For this review, use the dimensioned drawing (mm, ordinates from the lowest corner) and the shaded views. A direction names the side the tool comes from. Coordinates: 2 decimals unless noted, no trailing zeros. Loops run counter-clockwise (first coordinate to the right, second up) from the corner with the lowest first, then second, coordinate; pieces in that order, holes last.
1. Mouldability with a two-part tool opening along Y and no side actions: class the marked faces 3, 4 and 5 as pulls with the +Y half, pulls with the -Y half, needs draft (parallel to the pull), parting line crosses it, or undercut.
2. Take a section at C-C, the plane y = 19.05. State the section outline as (x, z) points (1 decimal), then the cut area to 3 significant figures.
3. Clearance check with flat-ended pins moving along their axes: P1, Ø8, axis at y = 17, z = 10, coming from the -X side (3 decimals); P2, Ø14.5, axis at y = 19.05, z = 12.7, coming from the +X side; P3, Ø6, axis at x = 27.5, y = 16, coming from the -Z side. State where each tip first meets the part, or that it passes through.
4. Take a section at A-A, the plane z = 30.48. State the section outline as (x, y) points.
5. Machinability: for the marked faces 1 and 2, which of the approach directions +Z, -Z, +X, -X, +Y, -Y give a long, thin tool a straight path to every point of the face, cutting with its end or side? Answer none if there is none.
6. Take a section at D-D, the plane y = 12.5. State the section outline as (x, z) points (3 decimals).
7. To check wall thickness, follow probe 1 along Y at (x, z) = (0.75, 30.48); probe 2 along Y at (x, z) = (19, 37); probe 3 along X at (y, z) = (19, 37). State the ranges of each line that lie inside material, in increasing order.
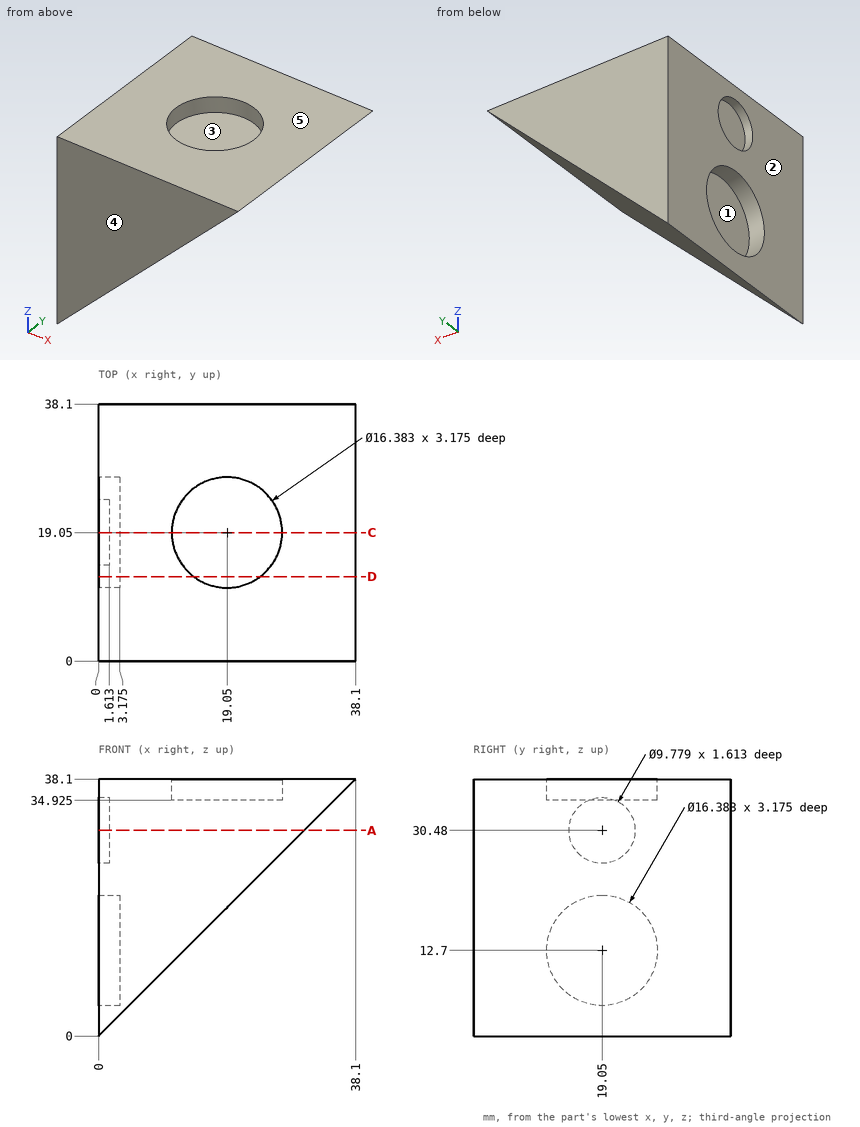
Results list:
1. face 3: undercut
1. face 4: pulls with the -Y half
1. face 5: needs draft
2. outline: (0, 0) - (38.1, 38.1) - (27.2, 38.1) - (27.2, 34.9) - (10.9, 34.9) - (10.9, 38.1) - (0, 38.1) - (0, 35.4) - (1.6, 35.4) - (1.6, 25.6) - (0, 25.6) - (0, 20.9) - (3.2, 20.9) - (3.2, 4.5) - (0, 4.5) - close
2. area: 606 mm2
3. P1: stops at x = 3.175
3. P2: stops at x = 19.95
3. P3: stops at z = 24.5
4. outline: (0, 0) - (30.48, 0) - (30.48, 38.1) - (0, 38.1) - (0, 23.94) - (1.61, 23.94) - (1.61, 14.16) - (0, 14.16) - close
5. face 1: -X
5. face 2: +Z, -Z, -X, +Y, -Y
6. outline: (0, 0) - (38.1, 38.1) - (23.969, 38.1) - (23.969, 34.925) - (14.131, 34.925) - (14.131, 38.1) - (0, 38.1) - (0, 17.619) - (3.175, 17.619) - (3.175, 7.781) - (0, 7.781) - close
7. probe 1: y = 0 to 14.16, 23.94 to 38.1
7. probe 2: y = 0 to 10.86, 27.24 to 38.1
7. probe 3: x = 0 to 10.86, 27.24 to 37
